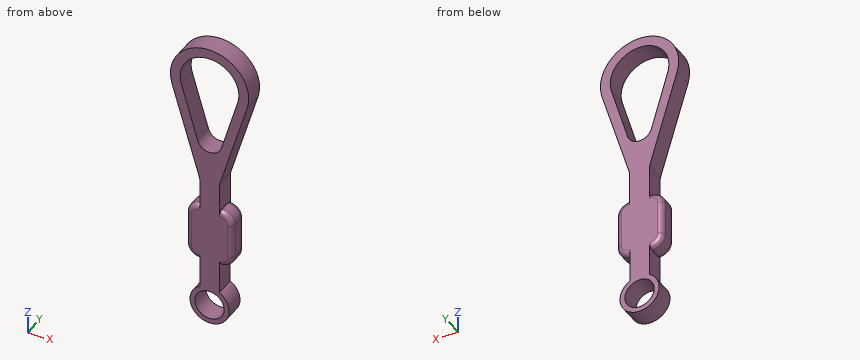
```python
from build123d import *

# Parameters (mm, degrees)
F0_R     = 1.5
F1_DEPTH = 2
F2_R     = 1.27
F3_R     = 0.508


with BuildPart() as f1:
    # F0 (on Front) → F1 (new body)
    with BuildSketch(Plane.XZ):
        with BuildLine():
            Line((-1, 4.7320508076), (-1, 1.7320508076))
            ThreePointArc((-1, 1.7320508076), (0, -2), (1, 1.7320508076))
            Line((1, 1.7320508076), (1, 4.7320508076))
            Line((1, 4.7320508076), (2.363858046, 4.7320508076))
            Line((2.363858046, 4.7320508076), (2.363858046, 10.7320508076))
            Line((2.363858046, 10.7320508076), (1.0033, 10.7320508076))
            Line((1.0033, 10.7320508076), (1.0033, 13.7320508076))
            Line((1.0033, 13.7320508076), (3.8344133108, 23.2630893134))
            ThreePointArc((3.8344133108, 23.2630893134), (-0.0012725797, 28.4020687255), (-3.8336878134, 23.2606497457))
            Line((-3.8336878134, 23.2606497457), (-0.9967, 13.7320508076))
            Line((-0.9967, 13.7320508076), (-0.9967, 10.7320508076))
            Line((-0.9967, 10.7320508076), (-2.363858046, 10.7320508076))
            Line((-2.363858046, 10.7320508076), (-2.363858046, 4.7320508076))
            Line((-2.363858046, 4.7320508076), (-1, 4.7320508076))
        make_face()
        Circle(F0_R, mode=Mode.SUBTRACT)
        with BuildLine():
            ThreePointArc((-2.8789812594, 23.5585839498), (0, 27.4020689279), (2.8789812594, 23.5585839498))
            Line((2.8789812594, 23.5585839498), (0, 13.7320508076))
            Line((0, 13.7320508076), (-2.8789812594, 23.5585839498))
        make_face(mode=Mode.SUBTRACT)
    extrude(amount=F1_DEPTH)

    # F2
    f2_edges = [f1.edges().sort_by_distance(p)[0] for p in [
        (2.363858, -1, 10.732051),
        (2.363858, -1, 4.732051),
        (-2.363858, -1, 10.732051),
        (-2.363858, -1, 4.732051),
        (0, -1, 13.732051),
        (1.0033, -1, 13.732051),
        (-0.9967, -1, 13.732051),
    ]]
    fillet(f2_edges, radius=F2_R)

    # F3
    f3_edges = [f1.edges().sort_by_distance(p)[0] for p in [
        (-1.991884, -2, 10.360076),
        (1.991884, -2, 10.360076),
        (2.363858, 0, 7.732051),
        (-2.363858, 0, 7.732051),
    ]]
    fillet(f3_edges, radius=F3_R)


solid = f1.part
```
Geometry check sheet. Reference: the model listing, model coordinates, mm. Round coordinates to 2 decimals unless told otherwise and drop trailing zeros. Order: outer loops, then holes, each group sorted by start corner. A loop starts at its lowest first (then second) coordinate and runs counter-clockwise, first axis right, second up. Notation, with made-up numbers: (57, 58.25) - (89, 58.25) arc R26 ccw to (89, 86.25) - close; hole circle Ø4 at (3, -26.5). An arc over 180 degrees is marked (long way). Use a Markdown table: item, result. Add a question column.
(1) Sectioned sample at A-A, the plane z = 0. Enter the section's corners in (x, y), and give its area (3 significant figures).
(2) Depth check by flat-ended pin: pin 1 (0.5 mm diameter, centred on y = -1, z = 7, fed in from +X); pin 2 (1 mm diameter, centred on y = -1.5, z = 3, fed in from -X); pin 3 (1 mm diameter, centred on y = -1, z = 11.5, fed in from +X); pin 4 (2.5 mm diameter, centred on x = 0, z = 0, fed in from +Y). Enter the tip coordinate at first touch or a pass-through.
(3) Sectioned sample at B-B, the plane x = 0. Enter the section's corners in (y, z).
(4) Sectioned sample at C-C, the plane y = -0.9. Enter the section's corners in (x, z).
(5) Material ranges on line 1 along Z through (x, y) = (0.25, -0.15); line 2 along X through (y, z) = (-1.9, 22); line 3 along X through (y, z) = (-0.1, 24.5), recorded low to high. Write a range as [from, to].
(6) Sectioned sample at D-D, the plane z = 8.5. Enter the section's corners in (x, y).
Answers below:
| question | item | result |
|---|---|---|
| 1 | outline | (-2, -2) - (-1.5, -2) - (-1.5, 0) - (-2, 0) - close; (1.5, -2) - (2, -2) - (2, 0) - (1.5, 0) - close |
| 1 | area | 2.00 mm² |
| 2 | pin 1 | x = 2.36 |
| 2 | pin 2 | x = -1 |
| 2 | pin 3 | x = 1 |
| 2 | pin 4 | through |
| 3 | outline | (-2, -2) - (0, -2) - (0, -1.5) - (-2, -1.5) - close; (-2, 1.5) - (0, 1.5) - (0, 16.98) - (-2, 16.98) - close; (-2, 27.4) - (0, 27.4) - (0, 28.4) - (-2, 28.4) - close |
| 4 | outline | (-3.83, 23.26) - (-1.05, 13.91) arc R1.27 cw to (-1, 13.55) - (-1, 10.73) - (-1.09, 10.73) arc R1.27 ccw to (-2.36, 9.46) - (-2.36, 6) arc R1.27 ccw to (-1.09, 4.73) - (-1, 4.73) - (-1, 1.73) arc R2 ccw (long way) to (1, 1.73) - (1, 4.73) - (1.09, 4.73) arc R1.27 ccw to (2.36, 6) - (2.36, 9.46) arc R1.27 ccw to (1.09, 10.73) - (1, 10.73) - (1, 13.55) arc R1.27 cw to (1.06, 13.91) - (3.83, 23.26) arc R4 ccw (long way) to start; hole (-2.88, 23.56) - (-1.22, 17.89) arc R1.27 ccw to (1.22, 17.89) - (2.88, 23.56) arc R3 ccw (long way) to start; hole circle Ø3 at (0, 0) |
| 5 | line 1 | [-1.98, -1.48], [1.48, 17], [27.39, 28.39] |
| 5 | line 2 | [-3.46, -2.42], [2.42, 3.46] |
| 5 | line 3 | [-4, -3], [3, 4] |
| 6 | outline | (-2.36, -1.49) arc R0.51 ccw to (-1.86, -2) - (1.86, -2) arc R0.51 ccw to (2.36, -1.49) - (2.36, -0.51) arc R0.51 ccw to (1.86, 0) - (-1.86, 0) arc R0.51 ccw to (-2.36, -0.51) - close |
